Source: CAD feature listing. Evaluate the final solid. Frame: model axes, mm. Face numbers are marked on the shaded views. A direction names the side the tool comes from. Coordinates: 2 decimals unless noted, no trailing zeros. Write each loop counter-clockwise with the first axis right and the second up, starting at its lowest first coordinate (ties: lowest second). Pieces come first, ordered by that corner, then holes. Notation, with made-up numbers: (-13, -8) - (-7, -8) arc R23 ccw to (-7, 0) - close; hole circle Ø7 at (55.25, 16). An arc over 180 degrees is marked (long way). One line per question, with ' | ' between items.
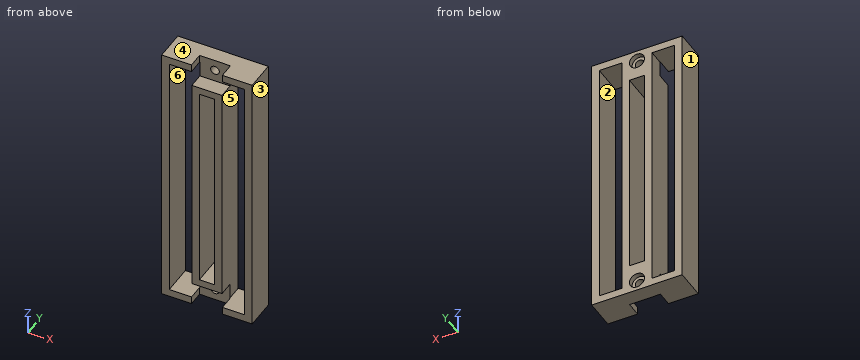
Autodesk Inventor part; units mm, degrees
ref_plane "YZ Plane" through (0, 0, 0) normal (1, 0, 0) x (0, 1, 0)
ref_plane "XZ Plane" through (0, 0, 0) normal (0, 1, 0) x (-1, 0, 0)
ref_plane "XY Plane" through (0, 0, 0) normal (0, 0, 1) x (1, 0, 0)
sketch "Sketch1" plane through (0, 0, 0) normal (0, 0, 1) x (1, 0, 0)
  line L0 (0, 0) -> (36, 0)
  line L1 (36, 0) -> (36, 12)
  line L2 (36, 12) -> (24, 12)
  line L3 (24, 12) -> (24, 22)
  line L4 (24, 22) -> (12, 22)
  line L5 (12, 22) -> (12, 12)
  line L6 (12, 12) -> (0, 12)
  line L7 (0, 12) -> (0, 0)
  dimension "d0" = 36
  dimension "d1" = 12
  dimension "d2" = 12
  dimension "d3" = 10
  dimension "d4" = 12
extrude "Extrusion1" add sketch "Sketch1" along normal blind 108
sketch "Sketch2" plane through (0, 0, 0) normal (0, -1, 0) x (1, 0, 0)
  circle A0 centre (18, 4.5) radius 1.725
  line L0 (0, 0) -> (36, 0)
  line L1 (36, 0) -> (36, 108)
  circle A1 centre (18, 103.5) radius 1.725
  line L2 (0, 108) -> (36, 108)
  dimension "d7" = 3.45
  dimension "d8" = 4.5
  dimension "d9" = 18
  dimension "d10" = 3.45
  dimension "d11" = 18
  dimension "d12" = 4.5
extrude "Extrusion2" cut sketch "Sketch2" against normal blind 20
sketch "Sketch3" plane through (12, 22, 0) normal (0, 1, 0) x (1, 0, 0)
  circle A0 centre (6, -4.5) radius 1.725
  circle A1 centre (6, -4.5) radius 3
  circle A2 centre (6, -103.5) radius 1.725
  circle A3 centre (6, -103.5) radius 3
  point P0 (-12, 0)
  dimension "d15" = 6
  dimension "d16" = 6
extrude "Extrusion3" cut sketch "Sketch3" against normal blind 2 contours A0 | A1 | A2 | A3
sketch "Sketch4" plane through (36, 0, 0) normal (1, 0, 0) x (0, 0, -1)
  line L0 (-108, 0) -> (-107.85, 0)
  line L1 (0, 0) -> (-108, 0)
  line L2 (-107.85, 0) -> (-107.85, 12)
  line L3 (0, 12) -> (-108, 12)
  line L4 (-108, 0) -> (-108, 12)
  line L5 (-108, 12) -> (-108, 0)
  line L6 (-108, 22) -> (-107.85, 22)
  line L7 (-107.85, 12) -> (-108, 12)
  line L8 (0, 0) -> (-0.15, 0)
  line L9 (-0.15, 0) -> (-0.15, 12)
  line L10 (-0.15, 12) -> (0, 12)
  line L11 (0, 12) -> (0, 0)
  line L12 (0, 22) -> (-0.15, 22)
  line L13 (-0.15, 12) -> (0, 12)
  dimension "d19" = 0.15
  dimension "d20" = 12
  dimension "d21" = 0.15
  dimension "d22" = 0.15
extrude "Extrusion4" cut sketch "Sketch4" against normal through all contours L4 L3 L2 L0 | L9 L3 L11 L1
sketch "Sketch5" plane through (24, 22, 108) normal (1, 0, 0) x (0, 0, -1)
  line L0 (108, -10) -> (108, 0)
  line L1 (108, 0) -> (0, 0)
  line L2 (108, -10) -> (107.85, -10)
  line L3 (107.85, -10) -> (107.85, 0)
  line L4 (107.85, 0) -> (108, 0)
  line L5 (108, 0) -> (108, -10)
  line L6 (0.15, -10) -> (0, -10)
  line L7 (0, -10) -> (0, 0)
  line L8 (0.15, -10) -> (0, -10)
  line L9 (0, -10) -> (0, 0)
  line L10 (0, 0) -> (0.15, 0)
  line L11 (0.15, 0) -> (0.15, -10)
  point P0 (108, -22)
  dimension "d25" = 0.15
extrude "Extrusion5" cut sketch "Sketch5" against normal through all
sketch "Sketch6" plane through (12, 22, 0.15) normal (0, 1, 0) x (1, 0, 0)
  point P0 (0, -107.7)
sketch "Sketch7" plane through (0, 0, 107.85) normal (0, -1, 0) x (1, 0, 0)
  line L0 (0, -107.7) -> (36, -107.7)
  line L1 (11.85, -107.7) -> (24.15, -107.7)
  line L2 (24.15, -107.7) -> (24.15, -98.55)
  line L3 (24.15, -98.55) -> (11.85, -98.55)
  line L4 (11.85, -98.55) -> (11.85, -107.7)
  line L5 (0, 0) -> (12, 0)
  line L6 (11.85, 0) -> (24.15, 0)
  line L7 (24.15, 0) -> (24.15, -9.15)
  line L8 (24.15, -9.15) -> (11.85, -9.15)
  line L9 (11.85, -9.15) -> (11.85, 0)
  line L10 (36, -107.7) -> (36, 0)
  point P0 (0, -107.85)
  dimension "d30" = 11.85
  dimension "d31" = 11.85
  dimension "d32" = 9.15
  dimension "d33" = 11.85
  dimension "d34" = 11.85
  dimension "d35" = 9.15
extrude "Extrusion6" cut sketch "Sketch7" against normal blind 6
sketch "Sketch8" plane through (36, 0, 0.15) normal (0, -1, 0) x (1, 0, 0)
  line L0 (-21, 95.7) -> (-15, 95.7)
  line L1 (-15, 95.7) -> (-15, 12)
  line L2 (-15, 12) -> (-21, 12)
  line L3 (-21, 12) -> (-21, 95.7)
  line L4 (-11.85, 0) -> (-24.15, 0)
  line L5 (0, 107.7) -> (-11.85, 107.7)
  line L6 (-24, 0) -> (-24, 107.7)
  line L7 (-12, 0) -> (-12, 107.7)
  point P0 (-36, -0.15)
  dimension "d38" = 12
  dimension "d39" = 12
  dimension "d40" = 3
  dimension "d41" = 3
extrude "Extrusion7" cut sketch "Sketch8" against normal through all
sketch "Sketch9" plane through (24, 12, 107.85) normal (0, 1, 0) x (1, 0, 0)
  line L0 (9, 3) -> (0, 3)
  line L1 (0, 3) -> (0, 104.7)
  line L2 (0, 104.7) -> (9, 104.7)
  line L3 (9, 104.7) -> (9, 3)
  line L4 (-12, 3) -> (-21, 3)
  line L5 (-21, 3) -> (-21, 104.7)
  line L6 (-21, 104.7) -> (-12, 104.7)
  line L7 (-12, 104.7) -> (-12, 3)
  line L8 (12, 0) -> (0.15, 0)
  line L9 (12, 107.7) -> (0, 107.7)
  line L10 (12, 107.7) -> (12, 0)
  line L11 (-24, 107.7) -> (-24, 0)
  line L12 (-12, 107.7) -> (-24, 107.7)
  line L13 (-24, 0) -> (-12, 0)
  line L14 (-12, 107.7) -> (-12, 0)
  line L15 (0, 107.7) -> (0, 0)
  point P0 (-24, 107.85)
  dimension "d44" = 3
  dimension "d45" = 3
  dimension "d46" = 3
  dimension "d47" = 3
  dimension "d48" = 3
  dimension "d49" = 3
  dimension "d50" = 0
  dimension "d51" = 0
extrude "Extrusion8" cut sketch "Sketch9" against normal through all contours L0 L1 L2 L3 | L4 L5 L6 L7
sketch "Sketch10" plane through (12, 0, 98.7) normal (0, -1, 0) x (1, 0, 0)
  line L0 (3, -86.55) -> (3, -2.85)
  line L1 (9, -2.85) -> (9, -86.55)
  line L2 (3, -2.85) -> (9, -2.85)
  line L3 (9, -2.85) -> (9, -86.55)
  line L4 (9, -86.55) -> (3, -86.55)
  line L5 (3, -86.55) -> (3, -2.85)
  line L6 (0, 0) -> (0, -89.4)
  line L7 (0, 0) -> (12, 0)
  line L8 (12, 0) -> (12, -89.4)
  line L9 (12, -89.4) -> (0, -89.4)
  line L10 (0, -89.4) -> (0, 0)
  line L11 (12, -89.4) -> (0, -89.4)
  line L12 (0, -89.4) -> (0, 0)
  line L13 (0, 0) -> (12, 0)
  line L14 (12, 0) -> (12, -89.4)
  point P0 (-12, -98.7)
sketch "Sketch11" plane through (24, 12, 0.15) normal (1, 0, 0) x (0, 0, -1)
  line L0 (-107.7, 0) -> (-107.7, 10)
  line L1 (0, 0) -> (-107.7, 0)
  line L2 (-107.7, 10) -> (0, 10)
  line L3 (0, 10) -> (0, 0)
  line L4 (0, 0) -> (-107.7, 0)
  line L5 (-107.7, 0) -> (-107.7, 10)
  point P0 (0.15, -12)
extrude "Extrusion9" cut sketch "Sketch11" against normal through all
sketch "Sketch12" plane through (0, 12, 107.85) normal (0, 1, 0) x (1, 0, 0)
  circle A0 centre (18, 103.35) radius 1.725
  circle A1 centre (18, 103.35) radius 3
  circle A2 centre (18, 4.35) radius 1.725
  circle A3 centre (18, 4.35) radius 3
  point P0 (0, 107.85)
  dimension "d56" = 6
  dimension "d57" = 6
extrude "Extrusion10" cut sketch "Sketch12" against normal blind 2
properties part number "topCenterBeam"
Item 1: Cut plane A-A on z = 103.5. Return loops of the section in (x, y) (3 decimals), and give its area (3 significant figures).
Check sheet entries:
outline: (0, 0) - (3, 0) - (3, 12) - (0, 12) - close; (12, 6) - (16.275, 6) - (16.275, 10) - (15, 10) - (15, 12) - (12, 12) - close; (19.725, 6) - (24, 6) - (24, 12) - (21, 12) - (21, 10) - (19.725, 10) - close; (33, 0) - (36, 0) - (36, 12) - (33, 12) - close | area: 118 mm²
Item 2: Mould query, pull axis Z, two halves, no side actions, for the marked faces 3, 4, 5 and 6. Classes: pulls with the +Z half, pulls with the -Z half, needs draft (parallel to the pull), parting line crosses it, or undercut.
Check sheet entries:
face 3: needs draft | face 4: pulls with the +Z half | face 5: undercut | face 6: undercut
Item 3: Pin query (flat end, axial travel): pin 1 Ø6.5 at (x, z) = (18.5, 3.5) entering from +Y; pin 2 Ø3 at (x, y) = (17.5, 3) entering from +Z; pin 3 Ø3 at (x, z) = (18, 104.5) entering from +Y; pin 4 Ø2 at (x, z) = (18, 4.5) entering from -Y. Return the tip coordinate at first contact, or that it passes through.
Check sheet entries:
pin 1: y = 12 | pin 2: z = 98.7 | pin 3: y = 10 | pin 4: through
Item 4: Ray query, line 1 along X through (y, z) = (0.5, 31.5); line 2 along X through (y, z) = (8.65, 4.5) (3 decimals); line 3 along Z through (x, y) = (18, 11.05). Return the intervals inside material, ascending. Write a range as [from, to].
Check sheet entries:
line 1: [0, 3], [12, 15], [21, 24], [33, 36] | line 2: [0, 3], [12, 16.275], [19.725, 24], [33, 36] | line 3: [0.15, 1.5], [7.5, 12.15], [95.85, 100.5], [106.5, 107.85]
Item 5: Cut plane B-B on y = 1. Return loops of the section in (x, z), and give its area (3 significant figures).
Check sheet entries:
outline: (0, 0.15) - (11.85, 0.15) - (11.85, 3.15) - (3, 3.15) - (3, 104.85) - (11.85, 104.85) - (11.85, 107.85) - (0, 107.85) - close; (12, 9.3) - (24, 9.3) - (24, 98.7) - (12, 98.7) - close; (24.15, 0.15) - (36, 0.15) - (36, 107.85) - (24.15, 107.85) - (24.15, 104.85) - (33, 104.85) - (33, 3.15) - (24.15, 3.15) - close; hole (15, 12.15) - (21, 12.15) - (21, 95.85) - (15, 95.85) - close | area: 1,320 mm²
Item 6: Access query for the marked faces 1 and 2. Directions: +Z, -Z, +X, -X, +Y, -Y. A direction counts if a zero-diameter tool reaches every point of the face in a straight line with its end or side. Return the directions, or none.
Check sheet entries:
face 1: +Z, -Z, -X, +Y, -Y | face 2: +Y, -Y
Item 7: Cut plane C-C on x = 18. Return loops of the section in (y, z) (3 decimals), and give its area (3 significant figures).
Check sheet entries:
outline: (0, 9.3) - (6, 9.3) - (6, 6.225) - (10, 6.225) - (10, 7.5) - (12, 7.5) - (12, 12.15) - (0, 12.15) - close; (0, 95.85) - (12, 95.85) - (12, 100.5) - (10, 100.5) - (10, 101.775) - (6, 101.775) - (6, 98.7) - (0, 98.7) - close; (6, 0.15) - (12, 0.15) - (12, 1.5) - (10, 1.5) - (10, 2.775) - (6, 2.775) - close; (6, 105.225) - (10, 105.225) - (10, 106.5) - (12, 106.5) - (12, 107.85) - (6, 107.85) - close | area: 127 mm²
Item 8: Cut plane D-D on x = 7.5. Return loops of the section in (y, z).
Check sheet entries:
outline: (0, 0.15) - (12, 0.15) - (12, 3.15) - (0, 3.15) - close; (0, 104.85) - (12, 104.85) - (12, 107.85) - (0, 107.85) - close
